Input: part model. Units: mm. Frame: model coordinates. Give positions to 0.01 mm unless a question says otherwise; leave off trailing zeros. Loops run counter-clockwise (first coordinate to the right, second up) from the corner with the lowest first, then second, coordinate; pieces in that order, holes last. Notation, with made-up numbers: (-24, 53.5) - (34, 53.5) arc R8 ccw to (34, 61.5) - close; hole circle Ø6 at (-39, 62). An arc over 180 degrees is marked (long way). One line per item, written item: value.
from build123d import *

# Parameters (mm, degrees)
F0_W     = 80
F0_H     = 80
F1_DEPTH = 2000
F2_W     = 25
F2_H     = 50
F3_DEPTH = 100


with BuildPart() as f1:
    # F0 (on Front) → F1 (new body)
    with BuildSketch(Plane.XZ):
        with BuildLine():
            Line((20.243097, 75.749835), (-59.756903, 75.749835))
            ThreePointArc((-59.756903, 75.749835), (-66.827971, 72.820903), (-69.756903, 65.749835))
            Line((-69.756903, 65.749835), (-69.756903, -14.250165))
            ThreePointArc((-69.756903, -14.250165), (-66.827971, -21.321233), (-59.756903, -24.250165))
            Line((-59.756903, -24.250165), (20.243097, -24.250165))
            ThreePointArc((20.243097, -24.250165), (27.314164, -21.321233), (30.243097, -14.250165))
            Line((30.243097, -14.250165), (30.243097, 65.749835))
            ThreePointArc((30.243097, 65.749835), (27.314164, 72.820903), (20.243097, 75.749835))
        make_face()
        with Locations((-19.756903, 25.749835)):
            Rectangle(F0_W, F0_H, mode=Mode.SUBTRACT)
    extrude(amount=F1_DEPTH)

    # F2 (on face) → F3 (cut)
    with BuildSketch(Plane(origin=(-69.756903, 0, 0), x_dir=(0, -1, 0), z_dir=(-1, 0, 0))):
        with Locations((42.5, 25)):
            Rectangle(F2_W, F2_H)
        with Locations((216.591, 25)):
            Rectangle(F2_W, F2_H)
        with Locations((390.682, 25)):
            Rectangle(F2_W, F2_H)
        with Locations((564.773, 25)):
            Rectangle(F2_W, F2_H)
        with Locations((1957.5, 25)):
            Rectangle(F2_W, F2_H)
        with Locations((738.864, 25)):
            Rectangle(F2_W, F2_H)
        with Locations((912.955, 25)):
            Rectangle(F2_W, F2_H)
        with Locations((1087.045, 25)):
            Rectangle(F2_W, F2_H)
        with Locations((1261.136, 25)):
            Rectangle(F2_W, F2_H)
        with Locations((1435.227, 25)):
            Rectangle(F2_W, F2_H)
        with Locations((1609.318, 25)):
            Rectangle(F2_W, F2_H)
        with Locations((1783.409, 25)):
            Rectangle(F2_W, F2_H)
    extrude(amount=-F3_DEPTH, mode=Mode.SUBTRACT)


solid = f1.part
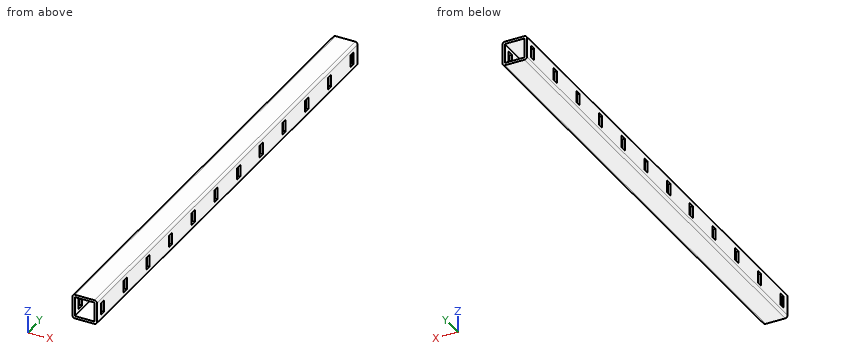
Item 1: Section C-C, the plane z = 27. Count the separate pieces of the cut face and the enclosed holes in it, and give its area (3 significant figures).
Verdict:
separate pieces: 26
enclosed holes: 0
area: 34,000 mm^2
Item 2: Pin query (flat end, axial travel): P1, Ø11, axis at x = -65.5, y = -40, coming from the +Z side; P2, Ø5, axis at x = -63, z = 18.5, coming from the +Y side; P3, Ø3, axis at x = -64.5, y = -1435, coming from the -Z side; P4, Ø3, axis at x = 27.5, y = -1082, coming from the +Z side. Return the tip coordinate at first contact, or that it passes through.
Verdict:
P1: stops at z = 75.75
P2: stops at y = 0
P3: stops at z = -23.71
P4: stops at z = 73.93
Item 3: Section A-A, the plane x = -3. Output: boundary loops of the cut face in (y, z), and give its area (3 significant figures).
Verdict:
outline: (-2000, -24.25) - (0, -24.25) - (0, -14.25) - (-2000, -14.25) - close; (-2000, 65.75) - (0, 65.75) - (0, 75.75) - (-2000, 75.75) - close
area: 40,000 mm^2
Item 4: Material intervals for L1, parallel to Z at x = -30, y = -717; L2, parallel to X at y = -446.5, z = 4; L3, parallel to Z at x = 26, y = -1107.5, sorted ascending.
Verdict:
L1: z = -24.25 to -14.25, 65.75 to 75.75
L2: x = -69.76 to -59.76, 20.24 to 30.24
L3: z = -22.43 to 73.93
Item 5: Section B-B, the plane y = -526.5. Output: boundary loops of the cut face in (x, z), and give its area (3 significant figures).
Verdict:
outline: (-69.76, -14.25) arc R10 ccw to (-59.76, -24.25) - (20.24, -24.25) arc R10 ccw to (30.24, -14.25) - (30.24, 65.75) arc R10 ccw to (20.24, 75.75) - (-59.76, 75.75) arc R10 ccw to (-69.76, 65.75) - close; hole (-59.76, -14.25) - (20.24, -14.25) - (20.24, 65.75) - (-59.76, 65.75) - close
area: 3,510 mm^2
